Source: CAD feature listing. Evaluate the final solid. Frame: model axes, mm. Face numbers are marked on the shaded views. A direction names the side the tool comes from. Round coordinates to 2 decimals unless told otherwise and drop trailing zeros. Write each loop counter-clockwise with the first axis right and the second up, starting at its lowest first coordinate (ties: lowest second). Pieces come first, ordered by that corner, then holes. Notation, with made-up numbers: M -36.75,-9.75 L -4.75,-9.75 A7 cw -4.75,3.25 Z; hole C 13,68.5 d1. An arc over 180 degrees is marked long. Answer in a Markdown table with one row per item. Add a question column.
Item 1: Cut plane A-A on y = 72.5. Return loops of the section in (x, z).
Item 2: Material intervals for probe 1 along Z at (x, y) = (39, 112); probe 2 along Z at (x, y) = (-31, 87.5); probe 3 along X at (y, z) = (-137, 8.75), sorted ascending.
Item 3: Set-up query: the marked faces 1 and 2. Return all of +Z, -Z, +X, -X, +Y, -Y with unobstructed straight access to the full face (end or side cutting, diameter ignored); none if empty.
Item 4: Contact query for flat-ended pins moving along their axis: pin 1 (12 mm diameter, centred on x = -39, y = 73.5, fed in from -Z); pin 2 (19 mm diameter, centred on x = 6.5, y = 64.5, fed in from -Z); pin 3 (11.5 mm diameter, centred on x = -8.5, y = -70.5, fed in from +Z); pin 4 (4 mm diameter, centred on y = -76, z = 21.5, fed in from +X). Output: stop coordinate, or through.
Item 5: Cut plane B-B on x = 9. Return loops of the section in (y, z).
Item 6: Cut plane C-C on x = -31. Return loops of the section in (y, z).
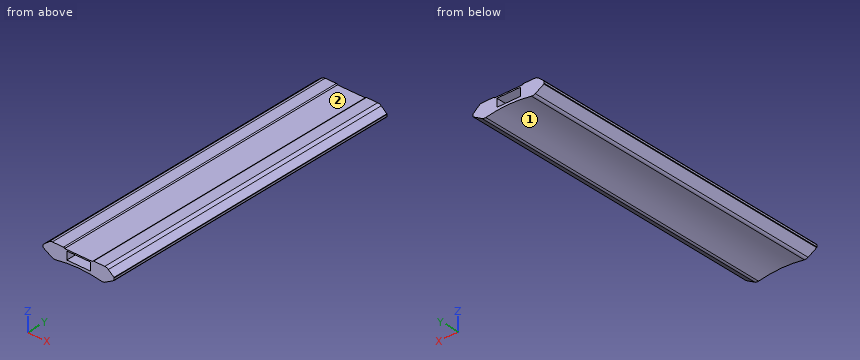
from build123d import *

# Parameters (mm, degrees)
F1_DEPTH    = 250
F2_W        = 38
F2_H        = 13
F3_DEPTH    = 250
F4_T1_DEPTH = 509.3674969976
F5_R        = 9
F6_R        = 1


# Not quite as in the source:
# - a fillet or chamfer that OpenCascade refuses, or shapes differently, is made with other operations: its cross-section is extruded or revolved along the edge and cut away or added


with BuildPart() as f1:
    # F0 (on Front) → F1 (new body, symmetric)
    with BuildSketch(Plane.XZ):
        with BuildLine():
            Line((22.5, 23.1507345177), (0, 23.1507345177))
            Line((0, 23.1507345177), (-22.5, 23.1507345177))
            Line((-22.5, 23.1507345177), (-22.5, 24.4507345177))
            Line((-22.5, 24.4507345177), (-45.5824640741, 24.4507345177))
            Line((-45.5824640741, 24.4507345177), (-57.5, 14.4507345177))
            Line((-57.5, 14.4507345177), (-57.5, 10.4507345177))
            Line((-57.5, 10.4507345177), (-40.1794919243, 0.4507345177))
            ThreePointArc((-40.1794919243, 0.4507345177), (0, 4.5282793762), (40.1794919243, 0.4507345177))
            Line((40.1794919243, 0.4507345177), (57.5, 10.4507345177))
            Line((57.5, 10.4507345177), (57.5, 14.4507345177))
            Line((57.5, 14.4507345177), (45.5824640741, 24.4507345177))
            Line((45.5824640741, 24.4507345177), (22.5, 24.4507345177))
            Line((22.5, 24.4507345177), (22.5, 23.1507345177))
        make_face()
    extrude(amount=F1_DEPTH, both=True)

    # F2 (on Front) → F3 (cut, symmetric)
    with BuildSketch(Plane.XZ):
        with Locations((0, 14.6507345177)):
            Rectangle(F2_W, F2_H)
    extrude(amount=F3_DEPTH, both=True, mode=Mode.SUBTRACT)

    # F4: fillet of radius 2 on 2 edges, made by hand

    # F4_s2 → F4_t1 (cut)
    with BuildSketch(Plane.XZ.offset(-254.6837484988)):
        with BuildLine():
            ThreePointArc((-24.3734993995, 24.4507345177), (-23.2333239744, 24.0939021903), (-22.5, 23.1507345177))
            Line((-22.5, 23.1507345177), (-22.5, 24.4507345177))
            Line((-22.5, 24.4507345177), (-24.3734993995, 24.4507345177))
        make_face()
        with BuildLine():
            ThreePointArc((24.3734993995, 24.4507345177), (23.2333239744, 24.0939021903), (22.5, 23.1507345177))
            Line((22.5, 23.1507345177), (22.5, 24.4507345177))
            Line((22.5, 24.4507345177), (24.3734993995, 24.4507345177))
        make_face()
    extrude(amount=F4_T1_DEPTH, mode=Mode.SUBTRACT)

    # F5
    f5_edges = [f1.edges().sort_by_distance(p)[0] for p in [
        (45.582464, 0, 24.450735),
        (40.179492, 0, 0.450735),
        (-45.582464, 0, 24.450735),
        (-40.179492, 0, 0.450735),
    ]]
    fillet(f5_edges, radius=F5_R)

    # F6
    f6_edges = [f1.edges().sort_by_distance(p)[0] for p in [
        (57.5, 0, 14.450735),
        (57.5, 0, 10.450735),
        (-57.5, 0, 14.450735),
        (-57.5, 0, 10.450735),
    ]]
    fillet(f6_edges, radius=F6_R)


solid = f1.part
Results below:
| question | item | result |
|---|---|---|
| 1 | outline | M -57.5,11.03 A1 ccw -57,10.16 L -43.1,2.14 A9 ccw -36.94,1.09 A200 cw 36.94,1.09 A9 ccw 43.1,2.14 L 57,10.16 A1 ccw 57.5,11.03 L 57.5,13.98 A1 ccw 57.14,14.75 L 48.09,22.35 A9 ccw 42.31,24.45 L 24.37,24.45 A2 ccw 22.5,23.15 L -22.5,23.15 A2 ccw -24.37,24.45 L -42.31,24.45 A9 ccw -48.09,22.35 L -57.14,14.75 A1 ccw -57.5,13.98 Z; hole M -19,8.15 L 19,8.15 L 19,21.15 L -19,21.15 Z |
| 2 | probe 1 | 0.94 to 24.45 |
| 2 | probe 2 | 2.11 to 24.45 |
| 2 | probe 3 | -54.55 to -19, 19 to 54.55 |
| 3 | face 1 | -Z, +Y, -Y |
| 3 | face 2 | +Z, +Y, -Y |
| 4 | pin 1 | z = 0.93 |
| 4 | pin 2 | z = 3.89 |
| 4 | pin 3 | z = 23.15 |
| 4 | pin 4 | x = 51.48 |
| 5 | outline | M -250,4.33 L 250,4.33 L 250,8.15 L -250,8.15 Z; M -250,21.15 L 250,21.15 L 250,23.15 L -250,23.15 Z |
| 6 | outline | M -250,2.11 L 250,2.11 L 250,24.45 L -250,24.45 Z |
